Part model, mm, in its own coordinate system. A direction names the side the tool comes from. Round coordinates to 2 decimals unless told otherwise and drop trailing zeros. Order: outer loops, then holes, each group sorted by start corner. A loop starts at its lowest first (then second) coordinate and runs counter-clockwise, first axis right, second up. Notation, with made-up numbers: (42.5, 16.25) -> (96.5, 16.25) arc R24 cw to (96.5, 48.25) -> close; hole circle Ø5 at (-8, 29). An arc over 180 degrees is marked (long way). Answer as a JSON object with one key per item and string values. Group by question number.
```python
from build123d import *

# Parameters (mm, degrees)
F0_W     = 200
F0_H     = 81
F1_DEPTH = 3
F2_W     = 200
F2_H     = 6
F2_H_2   = 5
F3_DEPTH = 1.8
F4_R     = 2


with BuildPart() as f1:
    # F0 (on Front) → F1 (new body)
    with BuildSketch(Plane.XZ):
        Rectangle(F0_W, F0_H)
    extrude(amount=F1_DEPTH)

    # F2 (on face) → F3 (cut)
    with BuildSketch(Plane.XZ.offset(3)):
        with Locations((0, 37.5)):
            Rectangle(F2_W, F2_H)
        with Locations((0, -38)):
            Rectangle(F2_W, F2_H_2)
    extrude(amount=-F3_DEPTH, mode=Mode.SUBTRACT)

    # F4
    f4_edges = [f1.edges().sort_by_distance(p)[0] for p in [
        (-100, -0.6, -40.5),
        (-100, -0.6, 40.5),
        (100, -0.6, -40.5),
        (100, -0.6, 40.5),
    ]]
    fillet(f4_edges, radius=F4_R)


solid = f1.part
```
Q1. Band-saw the part on B-B (y = -1.9). List the corners of the cut face in (x, z).
Q2. Band-saw the part on A-A (x = -84.5). List the corners of the cut face in (y, z), plus the area to 3 significant figures.
Q3. Which spindle directions (+Z, -Z, +X, -X, +Y, -Y) get a long thin tool onto all of the face, cutting with end or side? Do faces 1 (the flat face through (-1, -1.2, -38)), 2 (the flat face through (-1, 0, 1)), 3 (the flat face through (-1, -1.2, 38)). Say none if no direction does.
Q4. Wall check: line 1 (Z direction, x = 92, y = -1.4); line 2 (Y direction, x = -91.5, z = 35). Give the ranges that are in metal, low to high. Write a range as [from, to].
Q5. Drop flat-ended pins along their axis: pin 1 Ø2.5 at (x, z) = (42, -38.5) entering from -Y; pin 2 Ø1.4 at (x, y) = (-39, -2.5) entering from +Z. Give the stop position or say it passes through.
Completed:
{
 "1": {"outline": "(-100, -35.5) -> (100, -35.5) -> (100, 34.5) -> (-100, 34.5) -> close"},
 "2": {"outline": "(-3, -35.5) -> (-1.2, -35.5) -> (-1.2, -40.5) -> (0, -40.5) -> (0, 40.5) -> (-1.2, 40.5) -> (-1.2, 34.5) -> (-3, 34.5) -> close", "area": "223 mm2"},
 "3": {"face 1": "-Z, +X, -X, -Y", "face 2": "+Z, -Z, +X, -X, +Y", "face 3": "+Z, +X, -X, -Y"},
 "4": {"line 1": "[-35.5, 34.5]", "line 2": "[-1.2, 0]"},
 "5": {"pin 1": "y = -1.2", "pin 2": "z = 34.5"}
}
